The model under review builds one solid part; all positions refer to its coordinate system, in mm. A direction names the side the tool comes from. Round coordinates to 2 decimals unless told otherwise and drop trailing zeros. Loops run counter-clockwise (first coordinate to the right, second up) from the corner with the lowest first, then second, coordinate; pieces in that order, holes last. Notation, with made-up numbers: (39.5, 59.25) -> (65.5, 59.25) arc R14 cw to (65.5, 75.25) -> close; hole circle Ø2 at (28.25, 47.25). An arc over 180 degrees is marked (long way). Write each question's results on one line, items separated by ' | '. Start each with the question number.
Item 1: Clearance check with flat-ended pins moving along their axes: pin 1 Ø5.5 at (x, y) = (0, -12.5) entering from +Z; pin 2 Ø3 at (y, z) = (8.5, 2) entering from +X; pin 3 Ø3.5 at (x, y) = (-11, -29) entering from -Z; pin 4 Ø9 at (x, z) = (-4, 11) entering from +Y. State where each tip first meets the part, or that it passes through.
Item 2: For L1, parallel to Z at x = -5.5, y = -13; L2, parallel to Y at x = 0, z = 3.3; L3, parallel to Y at x = -8, z = 9, list the stretches that pass through material, from the lowest coordinate up. Write a range as from..to.
Item 3: We need section A-A (z = 3.5). Give the boundary of the cut face in (x, y).
Item 4: We need section D-D (y = -3). Give the boundary of the cut face in (x, z).
Item 5: We need section B-B (y = 6.25). Give the boundary of the cut face in (x, z), and give its area (3 significant figures).
Item 6: Tool access review of faces 4 (the flat face through (-11.4, -29.3, 5.5)), 5 (the flat face through (6, 6, 3)), 6 (the flat face through (0, -18, 11)): name each direction out of +Z, -Z, +X, -X, +Y, -Y from which nothing blocks a thin tool from reaching the whole face with its end or side.
Item 7: We need section C-C (z = 6). Give the boundary of the cut face in (x, y).
Item 8: Mouldability with a two-part tool opening along X and no side actions: class faces 1 (the cylindrical face through (-12.214, 5.185, 2.712)), 2 (the flat face through (12, -22, 8)), 3 (the flat face through (0, -24, 16.5)) as pulls with the +X half, pulls with the -X half, needs draft (parallel to the pull), parting line crosses it, or undercut.
from build123d import *

# Parameters (mm, degrees)
F0_R     = 1.75
F2_DEPTH = 5.5
F1_R     = 1.75
F3_DEPTH = 5.5
F4_R     = 3
F5_W     = 24
F5_H     = 12
F5_R     = 1.75
F6_DEPTH = 11


with BuildPart() as f2:
    # F0 (on Top) → F2 (new body)
    with BuildSketch(Plane.XY):
        with BuildLine():
            ThreePointArc((-12.0415945788, 13), (-12.4250770732, 12.9235481452), (-12.7499236717, 12.7058823529))
            ThreePointArc((-12.7499236717, 12.7058823529), (0, -18), (12.7499236717, 12.7058823529))
            ThreePointArc((12.7499236717, 12.7058823529), (12.4250770732, 12.9235481452), (12.0415945788, 13))
            Line((12.0415945788, 13), (7, 13))
            ThreePointArc((7, 13), (6.2928932188, 12.7071067812), (6, 12))
            Line((6, 12), (6, 0))
            ThreePointArc((6, 0), (0, -6), (-6, 0))
            Line((-6, 0), (-6, 12))
            ThreePointArc((-6, 12), (-6.2928932188, 12.7071067812), (-7, 13))
            Line((-7, 13), (-12.0415945788, 13))
        make_face()
        with Locations((-10.8253175473, -6.25)):
            Circle(F0_R, mode=Mode.SUBTRACT)
        with Locations((0, -12.5)):
            Circle(F0_R, mode=Mode.SUBTRACT)
        with Locations((10.8253175473, -6.25)):
            Circle(F0_R, mode=Mode.SUBTRACT)
        with Locations((-10.8253175473, 6.25)):
            Circle(F0_R, mode=Mode.SUBTRACT)
        with Locations((10.8253175473, 6.25)):
            Circle(F0_R, mode=Mode.SUBTRACT)
    extrude(amount=F2_DEPTH)

    # F1 (on Top) → F3 (join)
    with BuildSketch(Plane.XY):
        Polygon((12, -18), (0, -18), (-12, -18), (-12, -30), (12, -30), align=None)
        with Locations((-9, -24)):
            Circle(F1_R, mode=Mode.SUBTRACT)
        with Locations((9, -24)):
            Circle(F1_R, mode=Mode.SUBTRACT)
        with BuildLine():
            ThreePointArc((12, -13.416407865), (6.4227976159, -16.8151024613), (0, -18))
            Line((0, -18), (12, -18))
            Line((12, -18), (12, -13.416407865))
        make_face()
        with BuildLine():
            ThreePointArc((0, -18), (-6.4227976159, -16.8151024613), (-12, -13.416407865))
            Line((-12, -13.416407865), (-12, -18))
            Line((-12, -18), (0, -18))
        make_face()
    extrude(amount=F3_DEPTH)

    # F4
    f4_edges = [f2.edges().sort_by_distance(p)[0] for p in [
        (-12, -13.416408, 2.75),
        (-12, -30, 2.75),
        (12, -13.416408, 2.75),
        (12, -30, 2.75),
    ]]
    fillet(f4_edges, radius=F4_R)

    # F5 (on face) → F6 (join)
    with BuildSketch(Plane.XY.offset(5.5)):
        with Locations((0, -24)):
            Rectangle(F5_W, F5_H)
        with Locations((-9, -24)):
            Circle(F5_R, mode=Mode.SUBTRACT)
        with Locations((9, -24)):
            Circle(F5_R, mode=Mode.SUBTRACT)
    extrude(amount=F6_DEPTH)


solid = f2.part
Here are the results:
1) pin 1: stops at z = 5.5 | pin 2: stops at x = 16.58 | pin 3: stops at z = 0 | pin 4: stops at y = -18
2) L1: z = 0..5.5 | L2: y = -30..-14.25, -10.75..-6 | L3: y = -30..-25.44, -22.56..-18
3) outline: (-12.86, -12.6) arc R3 cw to (-12, -14.7) -> (-12, -27) arc R3 ccw to (-9, -30) -> (9, -30) arc R3 ccw to (12, -27) -> (12, -14.7) arc R3 cw to (12.86, -12.6) arc R18 ccw to (12.75, 12.71) arc R1 ccw to (12.04, 13) -> (7, 13) arc R1 ccw to (6, 12) -> (6, 0) arc R6 cw to (-6, 0) -> (-6, 12) arc R1 ccw to (-7, 13) -> (-12.04, 13) arc R1 ccw to (-12.75, 12.71) arc R18 ccw to start; hole circle Ø3.5 at (-10.83, -6.25); hole circle Ø3.5 at (-10.83, 6.25); hole circle Ø3.5 at (-9, -24); hole circle Ø3.5 at (0, -12.5); hole circle Ø3.5 at (9, -24); hole circle Ø3.5 at (10.83, -6.25); hole circle Ø3.5 at (10.83, 6.25)
4) outline: (-17.75, 0) -> (-5.2, 0) -> (-5.2, 5.5) -> (-17.75, 5.5) -> close; (5.2, 0) -> (17.75, 0) -> (17.75, 5.5) -> (5.2, 5.5) -> close
5) outline: (-16.88, 0) -> (-12.58, 0) -> (-12.58, 5.5) -> (-16.88, 5.5) -> close; (-9.08, 0) -> (-6, 0) -> (-6, 5.5) -> (-9.08, 5.5) -> close; (6, 0) -> (9.08, 0) -> (9.08, 5.5) -> (6, 5.5) -> close; (12.58, 0) -> (16.88, 0) -> (16.88, 5.5) -> (12.58, 5.5) -> close | area: 81.2 mm2
6) face 4: -Z, -X, -Y | face 5: +Z, -Z, +Y | face 6: +Z, +X, -X, +Y
7) outline: (-12, -30) -> (12, -30) -> (12, -18) -> (-12, -18) -> close; hole circle Ø3.5 at (-9, -24); hole circle Ø3.5 at (9, -24)
8) face 1: undercut | face 2: pulls with the +X half | face 3: needs draft
